```python
from build123d import *

# Parameters (mm, degrees)
SKETCH1_R               = 25
BOSS_EXTRUDE1_DEPTH     = 3
CUT_EXTRUDE1_DEPTH      = 36.482389998
CUT_EXTRUDE1_DEPTH_BACK = 36.482389998
SKETCH2_R               = 2.5


with BuildPart() as part:
    # Sketch1 → Boss-Extrude1 (new body)
    with BuildSketch(Plane.XY):
        Circle(SKETCH1_R)
        with BuildLine():
            Line((2.745911262, 19.401997604), (2.620473901, 4.376040727))
            ThreePointArc((2.620473901, 4.376040727), (3.650596033, 3.562269574), (4.438897848, 2.512528966))
            Line((4.438897848, 2.512528966), (19.534473328, 1.54333777))
            ThreePointArc((19.534473328, 1.54333777), (14.277143171, 13.42165126), (2.745911262, 19.401997604))
        make_face(mode=Mode.SUBTRACT)
        with BuildLine():
            Line((2.512528966, -4.438897848), (1.54333777, -19.534473328))
            ThreePointArc((1.54333777, -19.534473328), (13.42165126, -14.277143171), (19.401997604, -2.745911262))
            Line((19.401997604, -2.745911262), (4.376040727, -2.620473901))
            ThreePointArc((4.376040727, -2.620473901), (3.562269574, -3.650596033), (2.512528966, -4.438897848))
        make_face(mode=Mode.SUBTRACT)
        with BuildLine():
            Line((-4.438897848, -2.512528966), (-19.534473328, -1.54333777))
            ThreePointArc((-19.534473328, -1.54333777), (-14.277143171, -13.42165126), (-2.745911262, -19.401997604))
            Line((-2.745911262, -19.401997604), (-2.620473901, -4.376040727))
            ThreePointArc((-2.620473901, -4.376040727), (-3.650596033, -3.562269574), (-4.438897848, -2.512528966))
        make_face(mode=Mode.SUBTRACT)
        with BuildLine():
            Line((-2.512528966, 4.438897848), (-1.54333777, 19.534473328))
            ThreePointArc((-1.54333777, 19.534473328), (-13.42165126, 14.277143171), (-19.401997604, 2.745911262))
            Line((-19.401997604, 2.745911262), (-4.376040727, 2.620473901))
            ThreePointArc((-4.376040727, 2.620473901), (-3.562269574, 3.650596033), (-2.512528966, 4.438897848))
        make_face(mode=Mode.SUBTRACT)
    extrude(amount=BOSS_EXTRUDE1_DEPTH)

    # Sketch2 → Cut-Extrude1 (cut, two sides: drawn at the far end of the back side and taken through both)
    with BuildSketch(Plane(origin=(0, 0, 0), x_dir=(-1, 0, 0), z_dir=(0, 0, -1)).offset(-CUT_EXTRUDE1_DEPTH_BACK)):
        Circle(SKETCH2_R)
    extrude(amount=CUT_EXTRUDE1_DEPTH + CUT_EXTRUDE1_DEPTH_BACK, mode=Mode.SUBTRACT)


solid = part.part
```
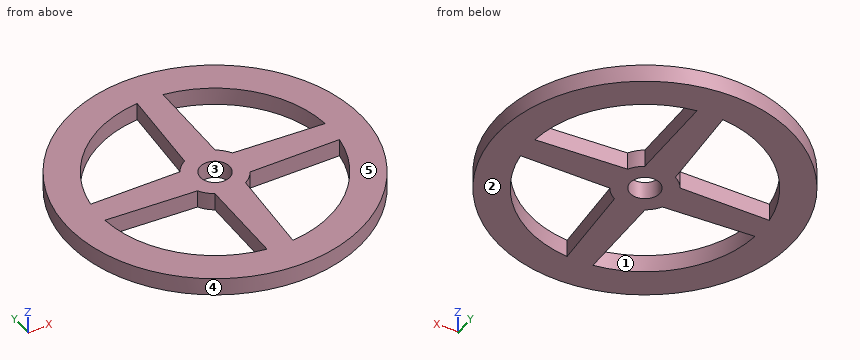
Input: part model. Units: mm. Frame: model coordinates. Face numbers are marked on the shaded views. A direction names the side the tool comes from. Round coordinates to 2 decimals unless told otherwise and drop trailing zeros. Write each loop counter-clockwise with the first axis right and the second up, starting at its lowest first coordinate (ties: lowest second). Pieces come first, ordered by that corner, then holes. Notation, with made-up numbers: M -17,10 L 28,10 A22 ccw 28,37 Z; hole C -6,40 d7. An arc over 180 degrees is marked long. Write each question's results on one line, items separated by ' | '.
Q1. Access query for the marked faces 1 and 2. Directions: +Z, -Z, +X, -X, +Y, -Y. A direction counts if a zero-diameter tool reaches every point of the face in a straight line with its end or side. Return the directions, or none.
Results:
face 1: +Z, -Z | face 2: -Z, +X, -X, +Y, -Y
Q2. Section query B-B (z = 1.8). Return loops of the section in (x, y).
Results:
outline: C 0,0 d50; hole M -19.53,-1.54 A19.6 ccw -2.75,-19.4 L -2.62,-4.38 A5.1 cw -4.44,-2.51 Z; hole M -19.4,2.75 L -4.38,2.62 A5.1 cw -2.51,4.44 L -1.54,19.53 A19.6 ccw Z; hole C 0,0 d5; hole M 1.54,-19.53 A19.6 ccw 19.4,-2.75 L 4.38,-2.62 A5.1 cw 2.51,-4.44 Z; hole M 2.62,4.38 A5.1 cw 4.44,2.51 L 19.53,1.54 A19.6 ccw 2.75,19.4 Z
Q3. Draft query along X for the marked faces 3, 4 and 5. Return one class per face: released by +X, released by -X, zero draft, split by the parting line, or undercut.
Results:
face 3: undercut | face 4: split by the parting line | face 5: zero draft
Q4. Line query: line 1 along Y through (x, z) = (0, 0.7); line 2 along Y through (x, z) = (-15, 2.15); line 3 along Y through (x, z) = (3.5, 0.4). Output: solid intervals per line, ascending.
Results:
line 1: y = -25 to -2.5, 2.5 to 25 | line 2: y = -20 to -12.61, -1.83 to 2.71, 12.61 to 20 | line 3: y = -24.75 to -19.28, -3.71 to 3.71, 19.28 to 24.75
Q5. Section query D-D (y = -14). Return loops of the section in (x, z), and give its area (3 significant figures).
Results:
outline: M -20.71,0 L -13.71,0 L -13.71,3 L -20.71,3 Z; M -2.7,0 L 1.9,0 L 1.9,3 L -2.7,3 Z; M 13.71,0 L 20.71,0 L 20.71,3 L 13.71,3 Z | area: 55.8 mm^2
Q6. Pin query (flat end, axial travel): P1, Ø4, axis at x = -6.5, y = -19, coming from the -Z side; P2, Ø4, axis at x = 0, y = 0, coming from the +Z side. Return the tip coordinate at first contact, or that it passes through.
Results:
P1: stops at z = 0 | P2: passes through
Q7. Section query A-A (x = 0). Return loops of the section in (y, z), and give its area (3 significant figures).
Results:
outline: M -25,0 L -2.5,0 L -2.5,3 L -25,3 Z; M 2.5,0 L 25,0 L 25,3 L 2.5,3 Z | area: 135 mm^2
